Autodesk Inventor part; units mm, degrees
ref_plane "Work Plane1" through (0, 0, 6) normal (0, 0, 1) x (1, 0, 0)
ref_plane "Work Plane3" through (14, 0, 12) normal (1, 0, 0) x (0, 0, -1)
ref_plane "YZ Plane" through (0, 0, 0) normal (1, 0, 0) x (0, 1, 0)
sketch "Sketch1" plane through (0, 0, 0) normal (0, 0, 1) x (1, 0, 0)
  line L0 (0, 0) -> (28, 0)
  line L1 (28, 0) -> (28, 13)
  line L2 (28, 13) -> (0, 13)
  line L3 (0, 13) -> (0, 0)
  circle A0 centre (7, 0) radius 4
  circle A1 centre (21, 0) radius 4
  point P0 (3, 0)
  point P1 (11, 0)
  point P2 (17, 0)
  point P3 (25, 0)
  dimension "d0" = 28
  dimension "d1" = 13
  dimension "d2" = 8
  dimension "d3" = 8
  dimension "d4" = 14
  dimension "d5" = 7
  dimension "d6" = 7
extrude "Extrusion1" add sketch "Sketch1" along normal blind 12 contours A1 L0 A0 L3 L2 L1
chamfer "Chamfer1" distance 6.5 angle 45 1 edges at (28, 13, 6)
sketch "Sketch2" plane through (0, 13, 12) normal (0, 1, 0) x (1, 0, 0)
  line L0 (0, 12) -> (0, 0)
  line L1 (0, 7.25) -> (11.5, 7.25)
  line L2 (11.5, 7.25) -> (11.5, 12)
  line L3 (21.5, 12) -> (0, 12)
  line L4 (17.5, 12) -> (17.5, 0)
  line L5 (11, 0) -> (17, 0)
  line L6 (0, 4.75) -> (11.5, 4.75)
  line L7 (11.5, 4.75) -> (11.5, 0)
  line L8 (11, 0) -> (3, 0)
  line L9 (11.5, 12) -> (17.5, 12)
  line L10 (25, 12) -> (17, 12)
  line L11 (17.5, 0) -> (11.5, 0)
  line L12 (0, 4.75) -> (0, 7.25)
  dimension "d12" = 6
  dimension "d13" = 2.5
  dimension "d14" = 11.5
extrude "Extrusion2" cut sketch "Sketch2" against normal blind 6 contours L1 L2 L3 L4 L11 L5 L7 L6 L0
fillet "Fillet1" radius 2 2 edges at (11.5, 10, 4.75) (11.5, 10, 7.25)
chamfer "Chamfer2" distance 0.5 angle 45 4 edges at (3, 0, 6) (11, 0, 6) (17, 0, 6) (25, 0, 6)
ref_plane "Work Plane1" through (0, 0, 6) normal (0, 0, 1) x (1, 0, 0)
ref_plane "Work Plane3" through (14, 0, 12) normal (1, 0, 0) x (0, 0, -1)
sketch "Sketch5" plane through (28, 0, 0) normal (0, -1, 0) x (1, 0, 0)
  circle A0 centre (3.5, 6) radius 1.5
  line L0 (-2.5, 0) -> (-2.5, 12)
  line L1 (-2.5, 0) -> (0, 0)
  line L2 (0, 0) -> (0, 12)
  line L3 (-2.5, 12) -> (0, 12)
  circle A1 centre (3.5, 6) radius 3.5
  line L4 (0, 0) -> (0, 12)
  line L5 (-6.5, 12) -> (0, 12)
  line L6 (0, 12) -> (5.9853, 12)
  line L7 (0, 0) -> (-6.5, 0)
  line L8 (0, 0) -> (5.9853, 0)
  line L9 (5.9853, 0) -> (7.7426, 1.7574)
  line L10 (5.9853, 12) -> (7.7426, 10.2426)
  circle A2 centre (3.5, 6) radius 6
  point P0 (-28, 0)
  point P1 (0, 6)
  dimension "d26" = 3
  dimension "d28" = 7
  dimension "d38" = 135
extrude "Extrusion3" add sketch "Sketch5" against normal blind 6.5 contours A0 | L2 A2 L8 | A1 | A2 L2 | L2 L6 A2 | A2 L9 L8 | L6 L10 A2 picked at (0.8638, 10.4147)
sketch "Sketch6" plane through (28, 6.5, 0) normal (0, 1, 0) x (1, 0, 0)
  arc A0 (7.7426, -10.2426) -> (7.7426, -1.7574) centre (3.5, -6) ccw
  point P0 (-28, 0)
hole "Hole1" at (31.5, 6.5, 6) direction (0, -1, 0) diameter 3.4 depth 8 countersink diameter 6.3 countersink angle 90
mirror "Mirror2" about plane through (14, 0, 12) normal (1, 0, 0) of "Extrusion3", "Hole1"
equation "\"d5\" = d6"
properties part number "Magnet Mount Lower"
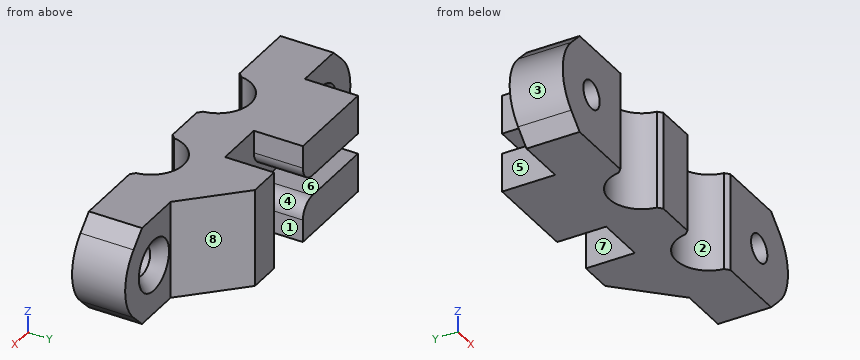
Can you work these out from the model? Positions are in its coordinate system, mm. Face numbers are marked on the shaded views. A direction names the side the tool comes from. Coordinates: 2 decimals unless noted, no trailing zeros. Order: outer loops, then holes, each group sorted by start corner. A loop starts at its lowest first (then second) coordinate and runs counter-clockwise, first axis right, second up. Notation, with made-up numbers: (-8.5, 80) -> (45.5, 80) arc R13 ccw to (45.5, 87) -> close; hole circle Ø4 at (70, 10.25). An arc over 180 degrees is marked (long way). Use one line per item in the form item = value.
Q1. I need wall thicknesses on L1, parallel to X at y = 2.5, z = 6; L2, parallel to Z at x = -3.5, y = 3.35; L3, parallel to X at y = 1, z = 4.75. Which ranges of each line are inside material? Lowest first, please.
From the geometry:
L1 = -9.5 to -5.2, -1.8 to 3.88, 10.12 to 17.88, 24.12 to 29.8, 33.2 to 37.5
L2 = 0 to 4.3, 7.7 to 12
L3 = -9.37 to -4.65, -2.35 to 3.13, 10.87 to 17.13, 24.87 to 30.35, 32.65 to 37.37
Q2. Will these pins go through, and if not, where does the flat tip stop? P1, Ø4, axis at x = 2, z = 3, coming from the -Y side; P2, Ø1.4, axis at y = 9, z = 1, coming from the +X side; P3, Ø2, axis at y = 10, z = 5.5, coming from the +X side; P4, Ø2, axis at x = 31.5, z = 6, coming from the -Y side.
From the geometry:
P1 = 0
P2 = 26.2
P3 = 25.5
P4 = through
Q3. Imagine slicing it at A-A, the plane y = 10.25. List the corners of the cut face in (x, z) for me.
From the geometry:
outline = (0, 0) -> (11.5, 0) -> (11.5, 2.75) arc R2 ccw to (9.5, 4.75) -> (0, 4.75) -> close; (0, 7.25) -> (9.5, 7.25) arc R2 ccw to (11.5, 9.25) -> (11.5, 12) -> (0, 12) -> close; (17.5, 0) -> (24.25, 0) -> (24.25, 12) -> (17.5, 12) -> close
Q4. We'd pull the mould along X, two halves only. Please class the marked faces 6, 7 and 8: released by +X, released by -X, zero draft, split by the parting line, or undercut.
From the geometry:
face_6 = zero draft
face_7 = undercut
face_8 = released by +X
Q5. Imagine slicing it at B-B, the plane x = -3.5. List the corners of the cut face in (y, z) for me, then the cut area to 3 significant figures.
From the geometry:
outline = (0, 0) -> (6.5, 0) -> (6.5, 2.85) -> (5.05, 4.3) -> (0, 4.3) -> close; (0, 7.7) -> (5.05, 7.7) -> (6.5, 9.15) -> (6.5, 12) -> (0, 12) -> close
area = 53.8 mm²
Q6. Imagine slicing it at D-D, the plane y = 1.5. List the corners of the cut face in (x, z) for me, then the cut area to 3 significant figures.
From the geometry:
outline = (-7.74, 1.76) -> (-5.99, 0) -> (3.29, 0) -> (3.29, 12) -> (-5.99, 12) -> (-7.74, 10.24) arc R6 ccw to start; (10.71, 0) -> (17.29, 0) -> (17.29, 12) -> (10.71, 12) -> close; (24.71, 0) -> (33.99, 0) -> (35.74, 1.76) arc R6 ccw to (35.74, 10.24) -> (33.99, 12) -> (24.71, 12) -> close; hole circle Ø3.4 at (-3.5, 6); hole circle Ø3.4 at (31.5, 6)
area = 340 mm²
Q7. Which directions (+Z, -Z, +X, -X, +Y, -Y) give clear straight access to the entire face, cutting with the end or side of a thin tool? Please do the marked faces 1, 2, 3, 4 and 5.
From the geometry:
face_1 = +Z, -Z, +Y
face_2 = +Z, -Z, -Y
face_3 = -X, +Y, -Y
face_4 = +Y
face_5 = +Z, -Z, -X, +Y
Q8. Imagine slicing it at C-C, the plane z = 6. Give the number of separate pieces and of enclosed holes in the cut face, then the cut area to 3 significant figures.
From the geometry:
separate_pieces = 3
enclosed_holes = 0
area = 262 mm²
